Geometry: final body of the model. Coordinates: model frame, mm. Face numbers are marked on the shaded views. A direction names the side the tool comes from. Give positions to 0.01 mm unless a question says otherwise; leave off trailing zeros. Write each loop counter-clockwise with the first axis right and the second up, starting at its lowest first coordinate (ties: lowest second). Pieces come first, ordered by that corner, then holes.
Q1. Section B-B (x = 0). Return the cut outline in (y, z).
Q2. Line query: line 1 (Z direction, x = -6.25, y = -1.75); line 2 (Z direction, x = -7, y = -6); line 3 (Y direction, x = 0, z = 17). Output: solid intervals per line, ascending.
Q3. Pin query (flat end, axial travel): pin 1 Ø10 at (x, z) = (-4.5, 19.5) entering from -Y; pin 2 Ø3 at (x, z) = (4.5, 19) entering from +Y; pin 3 Ø1 at (x, z) = (3, 17) entering from +Y. Return the tip coordinate at first contact, or that it passes through.
Q4. Section C-C (z = 21.25). Return the cut outline in (x, y).
Q5. Section A-A (y = 0). Return the cut outline in (x, z), plus the area to 3 significant figures.
Q6. Section D-D (x = 9). Return the cut outline in (y, z).
Q7. Reachability of the marked faces 1 and 2 from +Z, -Z, +X, -X, +Y, -Y: full face, straight path, thin tool, end or side. Return the list, or none.
Q8. Mould query, pull axis Z, two halves, no side actions, for the marked faces 3, 4 and 5. Classes: +Z half, -Z half, draft (parallel to the pull), parting line (faces both ways), or undercut.
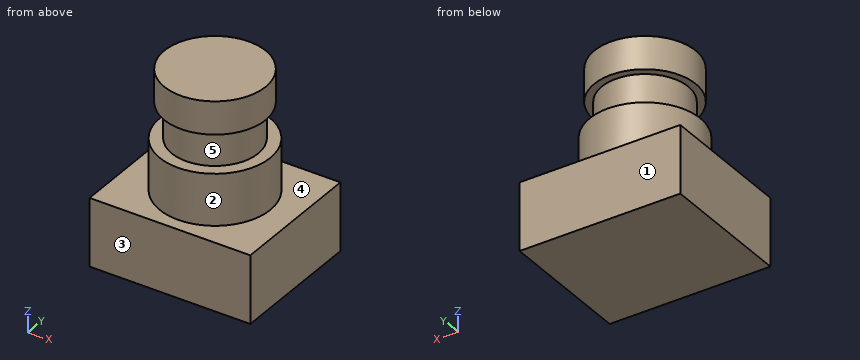
Autodesk Inventor part; units mm, degrees
ref_plane "YZ Plane" through (0, 0, 0) normal (1, 0, 0) x (0, 1, 0)
ref_plane "XZ Plane" through (0, 0, 0) normal (0, 1, 0) x (-1, 0, 0)
ref_plane "XY Plane" through (0, 0, 0) normal (0, 0, 1) x (1, 0, 0)
sketch "Sketch1" plane through (0, 0, 0) normal (0, 0, 1) x (1, 0, 0)
  line L0 (-11.25, 9.5) -> (11.25, 9.5)
  line L1 (11.25, 9.5) -> (11.25, -9.5)
  line L2 (11.25, -9.5) -> (-11.25, -9.5)
  line L3 (-11.25, -9.5) -> (-11.25, 9.5)
  point P0 (0, 0)
  point P1 (-11.25, 0)
  point P2 (0, 9.5)
  dimension "d0" = 19
  dimension "d1" = 22.5
extrude "Extrusion1" add sketch "Sketch1" along normal blind 9.5
sketch "Sketch2" plane through (0, 0, 9.5) normal (0, 0, 1) x (1, 0, 0)
  circle A0 centre (0, 0) radius 7.75
  dimension "d4" = 15.5
extrude "Extrusion2" add sketch "Sketch2" along normal blind 7.2
sketch "Sketch3" plane through (0, 0, 16.7) normal (0, 0, 1) x (1, 0, 0)
  circle A0 centre (0, 0) radius 6.05
  dimension "d7" = 12.1
extrude "Extrusion3" add sketch "Sketch3" along normal blind 5
sketch "Sketch4" plane through (0, 0, 21.7) normal (0, 0, 1) x (1, 0, 0)
  circle A0 centre (0, 0) radius 7.1
  dimension "d10" = 14.2
extrude "Extrusion4" add sketch "Sketch4" along normal blind 4.6
properties part number "Camera"
Computed:
1. outline: (-9.5, 0) - (9.5, 0) - (9.5, 9.5) - (7.75, 9.5) - (7.75, 16.7) - (6.05, 16.7) - (6.05, 21.7) - (7.1, 21.7) - (7.1, 26.3) - (-7.1, 26.3) - (-7.1, 21.7) - (-6.05, 21.7) - (-6.05, 16.7) - (-7.75, 16.7) - (-7.75, 9.5) - (-9.5, 9.5) - close
2. line 1: z = 0 to 16.7, 21.7 to 26.3
2. line 2: z = 0 to 9.5
2. line 3: y = -6.05 to 6.05
3. pin 1: stops at y = -7.74
3. pin 2: stops at y = 5.25
3. pin 3: stops at y = 7.3
4. outline: circle Ø12.1 at (0, 0)
5. outline: (-11.25, 0) - (11.25, 0) - (11.25, 9.5) - (7.75, 9.5) - (7.75, 16.7) - (6.05, 16.7) - (6.05, 21.7) - (7.1, 21.7) - (7.1, 26.3) - (-7.1, 26.3) - (-7.1, 21.7) - (-6.05, 21.7) - (-6.05, 16.7) - (-7.75, 16.7) - (-7.75, 9.5) - (-11.25, 9.5) - close
5. area: 451 mm2
6. outline: (-9.5, 0) - (9.5, 0) - (9.5, 9.5) - (-9.5, 9.5) - close
7. face 1: +Z, -Z, +X, -X, +Y
7. face 2: +Z
8. face 3: draft
8. face 4: +Z half
8. face 5: undercut
